Here's how the part is built. I have some questions about the finished solid (model axes, mm). Face numbers are marked on the shaded views. A direction names the side the tool comes from. Round coordinates to 2 decimals unless told otherwise and drop trailing zeros. Write each loop counter-clockwise with the first axis right and the second up, starting at its lowest first coordinate (ties: lowest second). Pieces come first, ordered by that corner, then holes. Notation, with made-up numbers: M -5,-2 L 20,-2 A17 cw 20,16 Z; hole C -18,-10.5 d8. An arc over 180 degrees is marked long. Use a Markdown table: item, result. Add a question column.
```python
from build123d import *

# Parameters (mm, degrees)
SKETCH1_W           = 32.4
SKETCH1_H           = 15
BOSS_EXTRUDE1_DEPTH = 10
SKETCH4_W           = 26.527336133
SKETCH4_H           = 10
CUT_EXTRUDE2_DEPTH  = 80
SKETCH5_R           = 2.75
CUT_EXTRUDE3_DEPTH  = 20
BOSS_EXTRUDE2_DEPTH = 10
BOSS_EXTRUDE3_DEPTH = 75.5
SKETCH9_W           = 43.572663867
SKETCH9_H           = 40.6
BOSS_EXTRUDE4_DEPTH = 9
FILLET1_R           = 6
SKETCH10_R          = 2.75
CUT_EXTRUDE4_DEPTH  = 20
SKETCH11_W          = 4
SKETCH11_H          = 7
CUT_EXTRUDE5_DEPTH  = 122
SKETCH12_R          = 3
BOSS_EXTRUDE5_DEPTH = 1.2
SKETCH13_R          = 2.7
BOSS_EXTRUDE6_DEPTH = 6.5
SKETCH14_R          = 1.5
CUT_EXTRUDE6_DEPTH  = 8
SKETCH15_R          = 4.2
CUT_EXTRUDE7_DEPTH  = 8
BOSS_EXTRUDE9_DEPTH = 6.5
SKETCH17_R          = 2.7
CUT_EXTRUDE8_DEPTH  = 8
SKETCH18_W          = 6
SKETCH18_H          = 12
CUT_EXTRUDE9_DEPTH  = 23
SKETCH19_R          = 6.5
CUT_EXTRUDE10_DEPTH = 23


with BuildPart() as part:
    # Sketch1 → Boss-Extrude1 (new body)
    with BuildSketch(Plane.XY):
        with Locations((-3.3, 7.5)):
            Rectangle(SKETCH1_W, SKETCH1_H)
        with Locations((-3.3, -7.5)):
            Rectangle(SKETCH1_W, SKETCH1_H)
        with Locations((-35.7, -7.5)):
            Rectangle(SKETCH1_W, SKETCH1_H)
        with Locations((-35.7, 7.5)):
            Rectangle(SKETCH1_W, SKETCH1_H)
    extrude(amount=BOSS_EXTRUDE1_DEPTH)

    # Sketch4 → Cut-Extrude2 (cut)
    with BuildSketch(Plane(origin=(0, 15, 0), x_dir=(1, 0, 0), z_dir=(0, 1, 0))):
        with Locations((-38.636331934, -5)):
            Rectangle(SKETCH4_W, SKETCH4_H)
    extrude(amount=-CUT_EXTRUDE2_DEPTH, mode=Mode.SUBTRACT)

    # Sketch5 → Cut-Extrude3 (cut)
    with BuildSketch(Plane.ZY.offset(25.372663867)):
        with Locations(Location((5, -8.5, 0), (0, 0, 270))):
            Circle(SKETCH5_R)
        with Locations(Location((5, 8.5, 0), (0, 0, 270))):
            Circle(SKETCH5_R)
    extrude(amount=-CUT_EXTRUDE3_DEPTH, mode=Mode.SUBTRACT)

    # Sketch7 → Boss-Extrude2 (add)
    with BuildSketch(Plane(origin=(0, 0, 0), x_dir=(-1, 0, 0), z_dir=(0, 0, -1))):
        Polygon((-12.9, -15.3), (-13.2, -15.3), (-13.2, 15.3), (-12.9, 15.3), (25.372663867, 15.3), (25.372663867, 15), (-12.9, 15), (-12.9, -15), (25.372663867, -15), (25.372663867, -15.3), align=None)
    extrude(amount=-BOSS_EXTRUDE2_DEPTH)

    # Sketch8 → Boss-Extrude3 (add)
    with BuildSketch(Plane(origin=(0, 0, 0), x_dir=(-1, 0, 0), z_dir=(0, 0, -1))):
        Polygon((25.372663867, 15.3), (25.372663867, 20.3), (-13.2, 20.3), (-18.2, 20.3), (-18.2, -15.3), (-18.2, -20.3), (-13.2, -20.3), (25.372663867, -20.3), (25.372663867, -15.3), (-13.2, -15.3), (-13.2, 15.3), align=None)
    extrude(amount=-BOSS_EXTRUDE3_DEPTH)

    # Sketch9 → Boss-Extrude4 (add)
    with BuildSketch(Plane.XY.offset(75.5)):
        with Locations((-3.586331933, 0)):
            Rectangle(SKETCH9_W, SKETCH9_H)
    extrude(amount=BOSS_EXTRUDE4_DEPTH)

    # Fillet1
    fillet1_edges = [part.edges().sort_by_distance(p)[0] for p in [
        (-3.586331933, 20.3, 84.5),
        (-3.586331933, -20.3, 84.5),
    ]]
    fillet(fillet1_edges, radius=FILLET1_R)

    # Sketch10 → Cut-Extrude4 (cut)
    with BuildSketch(Plane.ZY.offset(25.372663867)):
        with Locations(Location((80, 8.5, 0), (0, 0, 270))):
            Circle(SKETCH10_R)
        with Locations(Location((80, -8.5, 0), (0, 0, 270))):
            Circle(SKETCH10_R)
    extrude(amount=-CUT_EXTRUDE4_DEPTH, mode=Mode.SUBTRACT)

    # Sketch11 → Cut-Extrude5 (cut)
    with BuildSketch(Plane.XY.offset(84.5)):
        with Locations((-18.372663867, -8.5)):
            Rectangle(SKETCH11_W, SKETCH11_H)
        with Locations((-18.372663867, 8.5)):
            Rectangle(SKETCH11_W, SKETCH11_H)
    extrude(amount=-CUT_EXTRUDE5_DEPTH, mode=Mode.SUBTRACT)

    # Sketch12 → Boss-Extrude5 (add)
    with BuildSketch(Plane(origin=(0, 0, 0), x_dir=(-1, 0, 0), z_dir=(0, 0, -1))):
        with Locations((26.5, 0)):
            Circle(SKETCH12_R)
    extrude(amount=-BOSS_EXTRUDE5_DEPTH)

    # Sketch13 → Boss-Extrude6 (add)
    # profile 1 of 2: a face of its own
    with BuildSketch(Plane.XY):
        with BuildLine():
            ThreePointArc((-6.377852766, 30.969649026), (-3.586331933, 31.7), (-0.794811101, 30.969649026))
            Line((-0.794811101, 30.969649026), (18.2, 20.3))
            Line((18.2, 20.3), (-25.372663867, 20.3))
            Line((-25.372663867, 20.3), (-6.377852766, 30.969649026))
        make_face()
        with Locations(Location((-3.586331933, 26, 0), (0, 0, 180))):
            Circle(SKETCH13_R, mode=Mode.SUBTRACT)
    # profile 2 of 2: a face of its own
    with BuildSketch(Plane.XY):
        with BuildLine():
            Line((-25.372663867, -20.3), (-6.377852766, -30.969649026))
            ThreePointArc((-6.377852766, -30.969649026), (-3.586331933, -31.7), (-0.794811101, -30.969649026))
            Line((-0.794811101, -30.969649026), (18.2, -20.3))
            Line((18.2, -20.3), (-25.372663867, -20.3))
        make_face()
        with Locations(Location((-3.586331933, -26, 0), (0, 0, 180))):
            Circle(SKETCH13_R, mode=Mode.SUBTRACT)
    extrude(amount=BOSS_EXTRUDE6_DEPTH)

    # Sketch14 → Cut-Extrude6 (cut)
    with BuildSketch(Plane(origin=(0, 0, 0), x_dir=(-1, 0, 0), z_dir=(0, 0, -1))):
        with Locations((18.749186637, 17.9)):
            Circle(SKETCH14_R)
        with Locations((-11.57652277, 17.9)):
            Circle(SKETCH14_R)
        with Locations((-11.57652277, -17.9)):
            Circle(SKETCH14_R)
        with Locations((18.749186637, -17.9)):
            Circle(SKETCH14_R)
    extrude(amount=-CUT_EXTRUDE6_DEPTH, mode=Mode.SUBTRACT)

    # Sketch15 → Cut-Extrude7 (cut)
    with BuildSketch(Plane.ZY.offset(-13.2)):
        with Locations((62, 0)):
            Circle(SKETCH15_R)
    extrude(amount=-CUT_EXTRUDE7_DEPTH, mode=Mode.SUBTRACT)

    # Sketch16 → Boss-Extrude9 (add)
    with BuildSketch(Plane(origin=(0, 0, 0), x_dir=(-1, 0, 0), z_dir=(0, 0, -1))):
        with BuildLine():
            Line((-31.398424222, -4.876265107), (-18.2, -20.3))
            Line((-18.2, -20.3), (-18.2, 20.3))
            Line((-18.2, 20.3), (-31.398424222, 4.876265107))
            ThreePointArc((-31.398424222, 4.876265107), (-33.2, 0), (-31.398424222, -4.876265107))
        make_face()
    extrude(amount=-BOSS_EXTRUDE9_DEPTH)

    # Sketch17 → Cut-Extrude8 (cut)
    with BuildSketch(Plane(origin=(0, 0, 0), x_dir=(-1, 0, 0), z_dir=(0, 0, -1))):
        with Locations((-25.7, 0)):
            Circle(SKETCH17_R)
    extrude(amount=-CUT_EXTRUDE8_DEPTH, mode=Mode.SUBTRACT)

    # Sketch18 → Cut-Extrude9 (cut)
    with BuildSketch(Plane.XY.offset(84.5)):
        with Locations((-1.1, 0)):
            Rectangle(SKETCH18_W, SKETCH18_H)
    extrude(amount=-CUT_EXTRUDE9_DEPTH, mode=Mode.SUBTRACT)

    # Sketch19 → Cut-Extrude10 (cut)
    with BuildSketch(Plane(origin=(18.2, 0, 0), x_dir=(0, 0, -1), z_dir=(1, 0, 0))):
        with Locations((-62, 0)):
            Circle(SKETCH19_R)
    extrude(amount=-CUT_EXTRUDE10_DEPTH, mode=Mode.SUBTRACT)


solid = part.part
```
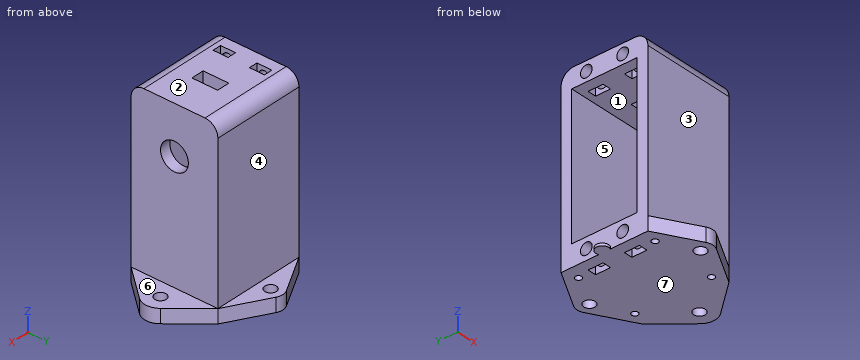
Item 1: Imagine slicing it at C-C on z = 43. List the corners of the cut face in (x, y) for me.
Item 2: Imagine slicing it at B-B on x = 25.7. List the corners of the cut face in (y, z) for me, plus the area to 3 significant figures.
Item 3: Imagine slicing it at A-A on y = 0. List the corners of the cut face in (x, z) for me, plus the area to 3 significant figures.
Item 4: I need wall thicknesses on probe 1 along Z at (x, y) = (-24.35, 8.5); probe 2 along Y at (x, z) = (-15.5, 54); probe 3 along Z at (x, y) = (9, 1.5). Which ranges of each line are inside material? Lowest first, please. Write a range as from..to.
Item 5: Imagine slicing it at D-D on y = 8.5. Count the separate pieces of the cut face and the enclosed holes in it, plus the area to 3 significant figures.
Item 6: If we mould it in two halves opening along Z, with no side actions, what happens to the marked faces 1, 2 and 3? For each: +Z half, -Z half, draft (parallel to the pull), parting line (faces both ways), or undercut.
Item 7: For pin 1 Ø5.5 at (y, z) = (-8, 78) entering from -X; pin 2 Ø1 at (y, z) = (5, 25.5) entering from -X; pin 3 Ø4.5 at (x, z) = (-19, 78.5) entering from -Y, each with a flat end and sliding along its axis, tell me the tip position at first contact or that it passes through.
Item 8: On a 3-axis mill with a long thin cutter (end or side, diameter ignored), from which of +Z, -Z, +X, -X, +Y, -Y can I reach the whole of each face in a straight line? I mean the marked faces 4, 5, 6 and 7. Say none if no direction works.
The answers:
| question | item | result |
|---|---|---|
| 1 | outline | M -25.37,-20.3 L 18.2,-20.3 L 18.2,20.3 L -25.37,20.3 L -25.37,15.3 L 13.2,15.3 L 13.2,-15.3 L -25.37,-15.3 Z |
| 2 | outline | M -11.54,0 L -2.7,0 L -2.7,6.5 L -11.54,6.5 Z; M 2.7,0 L 11.54,0 L 11.54,6.5 L 2.7,6.5 Z |
| 2 | area | 115 mm² |
| 3 | outline | M -29.5,0 L 23,0 L 23,6.5 L 18.2,6.5 L 18.2,55.5 L 13.2,55.5 L 13.2,10 L -25.37,10 L -25.37,1.2 L -29.5,1.2 Z; M -25.37,75.5 L -4.1,75.5 L -4.1,84.5 L -25.37,84.5 Z; M 1.9,75.5 L 13.2,75.5 L 13.2,68.5 L 18.2,68.5 L 18.2,84.5 L 1.9,84.5 Z; M 28.4,0 L 33.2,0 L 33.2,6.5 L 28.4,6.5 Z |
| 3 | area | 1,100 mm² |
| 4 | probe 1 | 0..2.25, 7.75..10, 75.5..77.25, 82.75..84.5 |
| 4 | probe 2 | -20.3..-15.3, 15.3..20.3 |
| 4 | probe 3 | 0..10, 75.5..84.5 |
| 5 | separate pieces | 5 |
| 5 | enclosed holes | 0 |
| 5 | area | 969 mm² |
| 6 | face 1 | undercut |
| 6 | face 2 | +Z half |
| 6 | face 3 | draft |
| 7 | pin 1 | x = -25.37 |
| 7 | pin 2 | x = 13.2 |
| 7 | pin 3 | y = -20.3 |
| 8 | face 4 | +Z, +X, -X, +Y |
| 8 | face 5 | -X |
| 8 | face 6 | +Z, +X, +Y, -Y |
| 8 | face 7 | -Z, +X, -X, +Y, -Y |
